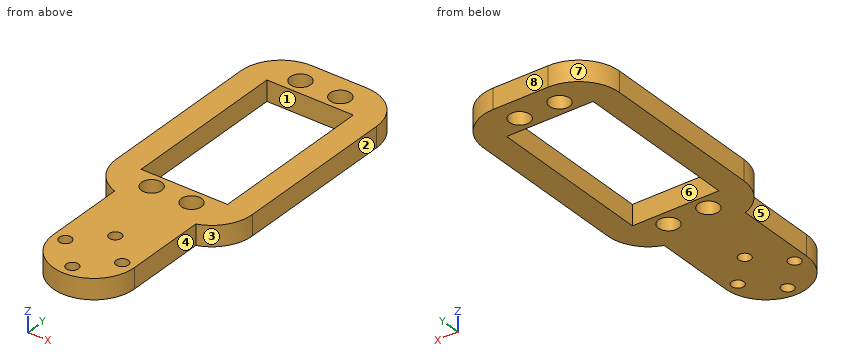
```python
from build123d import *

# Parameters (mm, degrees)
BOSS_EXTRUDE1_DEPTH = 5
SKETCH2_R           = 1.5
CUT_EXTRUDE1_DEPTH  = 10
SKETCH4_W           = 33.56
SKETCH4_H           = 60
BOSS_EXTRUDE2_DEPTH = 5
FILLET1_R           = 10
SKETCH3_R           = 2.5
SKETCH3_W           = 21.3
SKETCH3_H           = 41
CUT_EXTRUDE2_DEPTH  = 5


with BuildPart() as part:
    # Sketch1 → Boss-Extrude1 (new body)
    with BuildSketch(Plane.XY):
        with BuildLine():
            Line((10, 0), (10, 80))
            Line((10, 80), (-10, 80))
            Line((-10, 80), (-10, 0))
            ThreePointArc((-10, 0), (0, -10), (10, 0))
        make_face()
    extrude(amount=BOSS_EXTRUDE1_DEPTH)

    # Sketch2 → Cut-Extrude1 (cut)
    with BuildSketch(Plane.XY.offset(5)):
        with Locations((0, 7)):
            Circle(SKETCH2_R)
        with Locations((7, 0)):
            Circle(SKETCH2_R)
        with Locations((0, -7)):
            Circle(SKETCH2_R)
        with Locations((-7, 0)):
            Circle(SKETCH2_R)
    extrude(amount=-CUT_EXTRUDE1_DEPTH, mode=Mode.SUBTRACT)

    # Sketch4 → Boss-Extrude2 (add)
    with BuildSketch(Plane.XY.offset(5)):
        with Locations((0, 50)):
            Rectangle(SKETCH4_W, SKETCH4_H)
    extrude(amount=-BOSS_EXTRUDE2_DEPTH)

    # Fillet1
    # the kernel refuses this fillet: 10 mm, written as the material it takes off along each edge
    with BuildSketch(Plane(origin=(16.78, 80, 30), x_dir=(-1, 0, 0), z_dir=(0, 0, -1)), Plane(origin=(-16.78, 80, 30), x_dir=(0, -1, 0), z_dir=(0, 0, -1))) as fillet1_piece_1:
        with BuildLine():
            CenterArc((FILLET1_R, -FILLET1_R), FILLET1_R, 90, 90)
            Line((0, -FILLET1_R), (-FILLET1_R * 0.02, -FILLET1_R))
            Line((-FILLET1_R * 0.02, -FILLET1_R), (-FILLET1_R * 0.02, FILLET1_R * 0.02))
            Line((-FILLET1_R * 0.02, FILLET1_R * 0.02), (FILLET1_R, FILLET1_R * 0.02))
            Line((FILLET1_R, FILLET1_R * 0.02), (FILLET1_R, 0))
        make_face()
    extrude(amount=55, mode=Mode.SUBTRACT)
    with BuildSketch(Plane(origin=(16.78, 20, 28.668491714), x_dir=(0, 1, 0), z_dir=(0, 0, -1))) as fillet1_piece_2:
        with BuildLine():
            CenterArc((9.467396685, -10), FILLET1_R, 90, 71.216080389)
            Line((0, -6.78), (-0.189347934, -6.7156))
            ThreePointArc((-0.189347934, -6.7156), (-0.2, -3.39), (-0.2, 0))
            Line((-0.2, 0), (0, 0.2))
            Line((0, 0.2), (9.467396685, 0.2))
            Line((9.467396685, 0.2), (9.467396685, 0))
        make_face()
    extrude(amount=52.336983427, mode=Mode.SUBTRACT)
    with BuildSketch(Plane(origin=(-16.78, 20, 28.668491714), x_dir=(1, 0, 0), z_dir=(0, 0, -1))) as fillet1_piece_3:
        with BuildLine():
            CenterArc((10, -9.467396685), FILLET1_R, 108.783919611, 71.216080389)
            Line((0, -9.467396685), (-0.2, -9.467396685))
            Line((-0.2, -9.467396685), (-0.2, 0))
            Line((-0.2, 0), (0, 0.2))
            ThreePointArc((0, 0.2), (3.39, 0.2), (6.7156, 0.189347934))
            Line((6.7156, 0.189347934), (6.78, 0))
        make_face()
    extrude(amount=52.336983427, mode=Mode.SUBTRACT)

    # Sketch3 → Cut-Extrude2 (cut)
    with BuildSketch(Plane.XY.offset(5)):
        with Locations((4.6, 74.25)):
            Circle(SKETCH3_R)
        with Locations((-5.22372371, 74.25)):
            Circle(SKETCH3_R)
        with Locations((-5.22372371, 25.75)):
            Circle(SKETCH3_R)
        with Locations((4.6, 25.75)):
            Circle(SKETCH3_R)
        with Locations((0, 50)):
            Rectangle(SKETCH3_W, SKETCH3_H)
    extrude(amount=-CUT_EXTRUDE2_DEPTH, mode=Mode.SUBTRACT)


solid = part.part
```
Check sheet for the modelled part. Datum: model origin and axes. Units: mm. Face numbers are marked on the shaded views. A direction names the side the tool comes from. Round coordinates to 2 decimals unless told otherwise and drop trailing zeros. Order: outer loops, then holes, each group sorted by start corner. A loop starts at its lowest first (then second) coordinate and runs counter-clockwise, first axis right, second up. Notation, with made-up numbers: (83, 3) -> (139, 3) arc R19 ccw to (139, 13) -> close; hole circle Ø4 at (-30, 44.5). An arc over 180 degrees is marked (long way). Use CSV: the item, a comma, the result in double quotes.
(1) Tool access check on the marked faces 4, 5, 6, 7 and 8. Record the directions out of +Z, -Z, +X, -X, +Y, -Y that give a thin tool (end or side, any length) a straight path to the whole face; none if there is none.
Worked out:
face 4,"+Z, -Z, +X, -Y"
face 5,"+Z, -Z, -X, -Y"
face 6,"+Z, -Z"
face 7,"+Z, -Z, -X, +Y"
face 8,"+Z, -Z, +X, -X, +Y"
(2) Cross-section at C-C (y = 42). Record the boundary of the cut face in (x, z), and give its area (3 significant figures).
Worked out:
outline,"(-16.78, 0) -> (-10.65, 0) -> (-10.65, 5) -> (-16.78, 5) -> close; (10.65, 0) -> (16.78, 0) -> (16.78, 5) -> (10.65, 5) -> close"
area,"61.3 mm²"
(3) Cross-section at B-B (z = 3.1). Count the separate pieces of the cut face and the enclosed holes in it, and give its area (3 significant figures).
Worked out:
separate pieces,"1"
enclosed holes,"9"
area,"1,510 mm²"
(4) Cross-section at D-D (y = 25.75). Record the boundary of the cut face in (x, z), and give its area (3 significant figures).
Worked out:
outline,"(-16.06, 0) -> (-7.72, 0) -> (-7.72, 5) -> (-16.06, 5) -> close; (-2.72, 0) -> (2.1, 0) -> (2.1, 5) -> (-2.72, 5) -> close; (7.1, 0) -> (16.06, 0) -> (16.06, 5) -> (7.1, 5) -> close"
area,"111 mm²"
(5) Depth check by flat-ended pin: pin 1 (3 mm diameter, centred on y = 13.5, z = 0.5, fed in from -X); pin 2 (3.5 mm diameter, centred on x = 0, y = 7, fed in from +Z); pin 3 (2.5 mm diameter, centred on y = 11, z = 2, fed in from +X); pin 4 (1.5 mm diameter, centred on x = 10.5, z = 3, fed in from +Y). Enter the tip coordinate at first touch or a pass-through.
Worked out:
pin 1,"x = -10"
pin 2,"z = 5"
pin 3,"x = 10"
pin 4,"y = 79.55"
(6) Draft check along Y on the marked faces 1, 2 and 3. Enter one of: pulls with the +Y half, pulls with the -Y half, needs draft (parallel to the pull), parting line crosses it, or undercut.
Worked out:
face 1,"undercut"
face 2,"needs draft"
face 3,"pulls with the -Y half"
(7) Material ranges on line 1 along Y through (x, z) = (0, 2.45); line 2 along X through (y, z) = (52.5, 1.3); line 3 along Y through (x, z) = (4, 0.6), recorded low to high. Write a range as from..to.
Worked out:
line 1,"-10..-8.5, -5.5..5.5, 8.5..29.5, 70.5..80"
line 2,"-16.78..-10.65, 10.65..16.78"
line 3,"-9.17..23.32, 28.18..29.5, 70.5..71.82, 76.68..80"
(8) Cross-section at A-A (x = 0). Record the boundary of the cut face in (y, z).
Worked out:
outline,"(-10, 0) -> (-8.5, 0) -> (-8.5, 5) -> (-10, 5) -> close; (-5.5, 0) -> (5.5, 0) -> (5.5, 5) -> (-5.5, 5) -> close; (8.5, 0) -> (29.5, 0) -> (29.5, 5) -> (8.5, 5) -> close; (70.5, 0) -> (80, 0) -> (80, 5) -> (70.5, 5) -> close"
